```python
from build123d import *

# Parameters (mm, degrees)
PAD004_DEPTH    = 25
SKETCH011_R     = 1.375
POCKET007_DEPTH = 7
SKETCH012_R     = 2.75
POCKET008_DEPTH = 7
FILLET012_R     = 1
CHAMFER001_SIZE = 1


with BuildPart() as part:
    # Sketch008 (on XY_Plane003 of Origin006) → Pad004 (new body)
    with BuildSketch(Plane.XY):
        with BuildLine():
            ThreePointArc((0, 9.5), (-9.5, 0), (0, -9.5))
            Line((0, -9.5), (0, -16.99844))
            Line((-15, -16.99844), (0, -16.99844))
            Line((-15, -9.49844), (-15, -16.99844))
            Line((-6.483027, -9.49844), (-15, -9.49844))
            ThreePointArc((-5, 10.356158), (-11.468053, 0.856599), (-6.483027, -9.49844))
            Line((-5, 10.356158), (-5, 20.356158))
            Line((-5, 20.356158), (0, 20.356158))
            Line((0, 9.5), (0, 20.356158))
        make_face()
    extrude(amount=PAD004_DEPTH)

    # Sketch011 (on Face6 of Pad004) → Pocket007 (cut)
    with BuildSketch(Plane.XZ.offset(16.99844)):
        with Locations((-7.5, 12.5)):
            Circle(SKETCH011_R)
    extrude(amount=-POCKET007_DEPTH, mode=Mode.SUBTRACT)

    # Sketch012 (on Face1 of Pocket007) → Pocket008 (cut)
    with BuildSketch(Plane(origin=(-5, 0, 0), x_dir=(0, -1, 0), z_dir=(-1, 0, 0))):
        with Locations((-15.356158, 12.5)):
            Circle(SKETCH012_R)
    extrude(amount=-POCKET008_DEPTH, mode=Mode.SUBTRACT)

    # Fillet012
    fillet012_edges = [part.edges().sort_by_distance(p)[0] for p in [
        (-15, -13.24844, 0),
    ]]
    fillet(fillet012_edges, radius=FILLET012_R)

    # Chamfer001
    chamfer001_edges = [part.edges().sort_by_distance(p)[0] for p in [
        (-8.875, -16.99844, 12.5),
    ]]
    chamfer(chamfer001_edges, length=CHAMFER001_SIZE)


solid = part.part
```
Work out the finished part from the listing and answer in its coordinate system (mm). A direction names the side the tool comes from. Round coordinates to 2 decimals unless told otherwise and drop trailing zeros. Loops run counter-clockwise (first coordinate to the right, second up) from the corner with the lowest first, then second, coordinate; pieces in that order, holes last. Notation, with made-up numbers: (37.5, 73) -> (89.5, 73) arc R20 cw to (89.5, 83) -> close; hole circle Ø4 at (62.5, 14). An arc over 180 degrees is marked (long way). Write each question's results on one line, items separated by ' | '. Start each with the question number.
1. Given pin 1 Ø5 at (y, z) = (16, 9) entering from -X; pin 2 Ø1 at (y, z) = (-3, 3) entering from +X; pin 3 Ø1.6 at (x, z) = (-7.5, 12.5) entering from +Y, each flat-ended and moving along its own axis, determine where each tip first touches the part or whether it passes through.
2. Section B-B (y = -11) is taken. Determine the outline of the cut face in (x, z) (3 decimals), plus the area to 3 significant figures.
3. Section D-D (y = 17) is taken. Determine the outline of the cut face in (x, z).
4. Find the intervals of material crossed by probe 1 along Z at (x, y) = (-7.5, -14.25) (3 decimals); probe 2 along Y at (x, z) = (-6.75, 16); probe 3 along Y at (x, z) = (-4.25, 10.5), in increasing order. Write a range as from..to.
5. A tool of negligible diameter and unlimited length cuts with its end or side. For faces 4 (the face through (-5, 15.3, 9.5)), 5 (the face through (0, -13, 12)), 6 (the face through (-8, -9.998, 13)), from which of +Z, -Z, +X, -X, +Y, -Y can it reach the whole face along a straight path? Write none if from no direction.
6. Section C-C (x = -7.5) is taken. Determine the outline of the cut face in (y, z) (3 decimals), plus the area to 3 significant figures.
7. For a pull along X with two mould halves and no side action, classify faces 1 (the face through (-8.874, -13.04, 12.56)), 2 (the face through (-11.454, 1.025, 12.325)), 3 (the face through (-11, -9.498, 12)) as +X half, -X half, draft (parallel to the pull), parting line (faces both ways), or undercut.
8. Section A-A (z = 7) is taken. Determine the outline of the cut face in (x, y).
Evaluation:
1) pin 1: stops at x = -5 | pin 2: stops at x = -8.83 | pin 3: stops at y = 9.35
2) outline: (-15, 1) arc R1 ccw to (-14, 0) -> (0, 0) -> (0, 25) -> (-15, 25) -> close; hole circle Ø2.75 at (-7.5, 12.5) | area: 369 mm2
3) outline: (-5, 0) -> (0, 0) -> (0, 10.3) -> (-5, 10.3) -> close; (-5, 14.7) -> (0, 14.7) -> (0, 25) -> (-5, 25) -> close
4) probe 1: z = 0..11.125, 13.875..25 | probe 2: y = -17..-9.5, -9.31..-6.68, 6.68..9.31 | probe 3: y = -17..-8.5, 8.5..13.47, 17.24..20.36
5) face 4: +Z, -Z, -X, +Y | face 5: +Z, -Z, +X, +Y, -Y | face 6: -Y
6) outline: (-16.998, 0) -> (-9.498, 0) -> (-9.498, 25) -> (-16.998, 25) -> (-16.998, 14.875) -> (-15.998, 13.875) -> (-9.998, 13.875) -> (-9.998, 11.125) -> (-15.998, 11.125) -> (-16.998, 10.125) -> close; (-8.718, 0) -> (-5.831, 0) -> (-5.831, 25) -> (-8.718, 25) -> close; (5.831, 0) -> (8.718, 0) -> (8.718, 25) -> (5.831, 25) -> close | area: 312 mm2
7) face 1: undercut | face 2: -X half | face 3: draft
8) outline: (-15, -17) -> (0, -17) -> (0, -9.5) arc R9.5 cw to (0, 9.5) -> (0, 20.36) -> (-5, 20.36) -> (-5, 10.36) arc R11.5 ccw to (-6.48, -9.5) -> (-15, -9.5) -> close
